from build123d import *

# Parameters (mm, degrees)
SKETCH3_R           = 3.739985504
BOSS_EXTRUDE1_DEPTH = 2
SKETCH4_W           = 20.9095389
SKETCH4_H           = 29.780418306
BOSS_EXTRUDE2_DEPTH = 7


with BuildPart() as part:
    # Sketch3 → Boss-Extrude1 (new body)
    with BuildSketch(Plane.XY):
        with BuildLine():
            Line((-60.167323843, -17.670722848), (-60.167323843, -27.522824769))
            Line((-60.167323843, -27.522824769), (-39.257784943, -27.522824769))
            Line((-39.257784943, -27.522824769), (-39.257784943, 2.257593537))
            Line((-39.257784943, 2.257593537), (-60.167323843, 2.257593537))
            Line((-60.167323843, 2.257593537), (-60.167323843, -7.594508384))
            ThreePointArc((-60.167323843, -7.594508384), (-65.205431076, -12.632615616), (-60.167323843, -17.670722848))
        make_face()
        with Locations((-60.167323843, -12.632615616)):
            Circle(SKETCH3_R, mode=Mode.SUBTRACT)
    extrude(amount=BOSS_EXTRUDE1_DEPTH)

    # Sketch4 → Boss-Extrude2 (add)
    with BuildSketch(Plane.XY.offset(2)):
        with Locations((-49.712554393, -12.632615616)):
            Rectangle(SKETCH4_W, SKETCH4_H)
    extrude(amount=BOSS_EXTRUDE2_DEPTH)


solid = part.part
The listing builds one solid part. Answer for the finished solid, in the listing's coordinates (mm). A direction names the side the tool comes from. Round coordinates to 2 decimals unless told otherwise and drop trailing zeros. Order: outer loops, then holes, each group sorted by start corner. A loop starts at its lowest first (then second) coordinate and runs counter-clockwise, first axis right, second up. Notation, with made-up numbers: M 23.5,-1 L 66.5,-1 A12 cw 66.5,21 Z; hole C -17.75,29 d3. An arc over 180 degrees is marked long. Answer in a Markdown table with one row per item. Add a question column.
1) The part is cut by section B-B on x = -63. Determine the outline of the cut face in (y, z).
2) Determine the mould class of faces 1 (the face through (-50, -12, 9)), 2 (the face through (-50, -12, 0)), 3 (the face through (-39.258, -13, 4)) for opening direction Z: pulls with the +Z half, pulls with the -Z half, needs draft (parallel to the pull), parting line crosses it, or undercut.
3) Which of the six approach directions +Z, -Z, +X, -X, +Y, -Y give full straight-line access (tool end or side, diameter ignored) to faces 4 (the face through (-64.4, -12.6, 2)), 5 (the face through (-50, 2.258, 4)), 6 (the face through (-59, -13, 2))?
4) Consider line 1 along Z through (x, y) = (-58.25, -15.5); line 2 along X through (y, z) = (-11.5, 5.5). Determine where each line is inside the solid, lowest interval first. Write a range as from..to.
5) The part is cut by section A-A on y = -15. Determine the outline of the cut face in (x, z).
6) The part is cut by section D-D on x = -59.5. Determine the outline of the cut face in (y, z), plus the area to 3 significant figures.
7) The part is cut by section C-C on z = 1.25. Determine the outline of the cut face in (x, y).
8) Flat-ended cylindrical pins translate along their axes: pin 1 Ø3 at (x, y) = (-58, -13) entering from -Z; pin 2 Ø4.5 at (y, z) = (-19, 4.5) entering from -X. Find the tip coordinate at first contact, or state that the pin passes through.
Findings below:
| question | item | result |
|---|---|---|
| 1 | outline | M -16.8,0 L -15.07,0 L -15.07,2 L -16.8,2 Z; M -10.19,0 L -8.47,0 L -8.47,2 L -10.19,2 Z |
| 2 | face 1 | pulls with the +Z half |
| 2 | face 2 | pulls with the -Z half |
| 2 | face 3 | needs draft |
| 3 | face 4 | +Z, -X, +Y, -Y |
| 3 | face 5 | +Z, -Z, +X, -X, +Y |
| 3 | face 6 | -Z |
| 4 | line 1 | z = 2..9 |
| 4 | line 2 | x = -60.17..-39.26 |
| 5 | outline | M -64.61,0 L -63.06,0 L -63.06,2 L -64.61,2 Z; M -60.17,2 L -57.27,2 L -57.27,0 L -39.26,0 L -39.26,9 L -60.17,9 Z |
| 6 | outline | M -27.52,0 L -16.31,0 L -16.31,2 L -8.95,2 L -8.95,0 L 2.26,0 L 2.26,9 L -27.52,9 Z |
| 6 | area | 253 mm² |
| 7 | outline | M -60.17,-27.52 L -39.26,-27.52 L -39.26,2.26 L -60.17,2.26 L -60.17,-7.59 A5.04 ccw -60.17,-17.67 Z; hole C -60.17,-12.63 d7.48 |
| 8 | pin 1 | stops at z = 2 |
| 8 | pin 2 | stops at x = -60.17 |
